Could you check a few things on this model? Use its own coordinates, in mm. Give positions to 0.01 mm unless a question says otherwise; leave off trailing zeros. Loops run counter-clockwise (first coordinate to the right, second up) from the corner with the lowest first, then second, coordinate; pieces in that order, holes last. Notation, with made-up numbers: M 45.5,-35.75 L 82.5,-35.75 A21 cw 82.5,-28.75 Z; hole C -21,63 d8. An arc over 180 degrees is marked long. Return JSON: item names as keys, results as strings. Group by question number.
1. If we section it at A-A (y = 1.45): Write out the boundary of the cut face in (x, z).
2. If we section it at C-C (z = -87): Write out the boundary of the cut face in (x, y).
3. For pin 1 (2 mm diameter, centred on x = 8, z = 0, fed in from +Y); pin 2 (1.5 mm diameter, centred on y = 1.5, z = -9.5, fed in from +X); pin 3 (6 mm diameter, centred on x = -32, z = -51.5, fed in from -Y), each with a flat end and sliding along its axis, tell me the tip position at first contact or that it passes through.
4. Please list where these lines run through material, in increasing order: line 1 (Z direction, x = 4, y = 2.15); line 2 (Z direction, x = -4, y = 0.75); line 3 (Z direction, x = -8, y = 0.85).
5. If we section it at B-B (x = 120): Write out the boundary of the cut face in (y, z).
```python
from build123d import *

# Parameters (mm, degrees)
SKETCH1_R           = 150
BOSS_EXTRUDE1_DEPTH = 3
SKETCH3_R           = 1.25
CUT_EXTRUDE1_DEPTH  = 10


with BuildPart() as part:
    # Sketch1 → Boss-Extrude1 (new body)
    with BuildSketch(Plane(origin=(0, 0, 0), x_dir=(1, 0, 0), z_dir=(0, 1, 0))):
        Circle(SKETCH1_R)
    extrude(amount=BOSS_EXTRUDE1_DEPTH)

    # Sketch3 → Cut-Extrude1 (cut)
    with BuildSketch(Plane.XZ):
        with Locations((8, 0)):
            Circle(SKETCH3_R)
        with Locations((4, 6.92820323)):
            Circle(SKETCH3_R)
        with Locations((4, -6.92820323)):
            Circle(SKETCH3_R)
        with Locations((-4, 6.92820323)):
            Circle(SKETCH3_R)
        with Locations((-8, 0)):
            Circle(SKETCH3_R)
    extrude(amount=-CUT_EXTRUDE1_DEPTH, mode=Mode.SUBTRACT)


solid = part.part
```
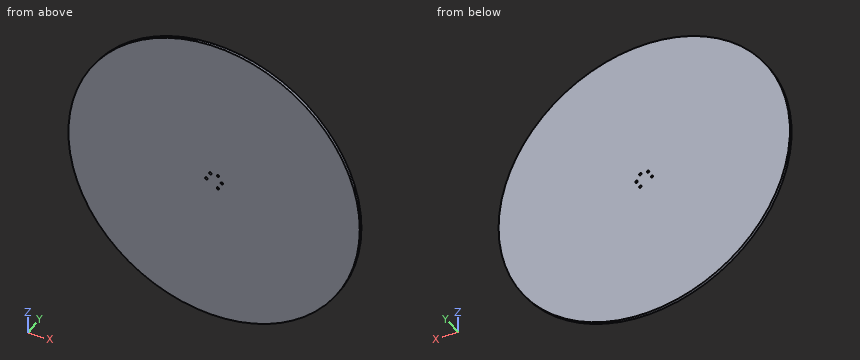
Answer:
{
 "1": {"outline": "C 0,0 d300; hole C -8,0 d2.5; hole C -4,6.93 d2.5; hole C 4,-6.93 d2.5; hole C 4,6.93 d2.5; hole C 8,0 d2.5"},
 "2": {"outline": "M -122.19,0 L 122.19,0 L 122.19,3 L -122.19,3 Z"},
 "3": {"pin 1": "passes through", "pin 2": "stops at x = 149.74", "pin 3": "stops at y = 0"},
 "4": {"line 1": "z = -149.95 to -8.18, -5.68 to 5.68, 8.18 to 149.95", "line 2": "z = -149.95 to 5.68, 8.18 to 149.95", "line 3": "z = -149.79 to -1.25, 1.25 to 149.79"},
 "5": {"outline": "M 0,-90 L 3,-90 L 3,90 L 0,90 Z"}
}
